Read the model definition and answer for the solid it produces. Units are mm, in the model's axes. A direction names the side the tool comes from. Coordinates: 2 decimals unless noted, no trailing zeros. Loops run counter-clockwise (first coordinate to the right, second up) from the corner with the lowest first, then second, coordinate; pieces in that order, holes last. Notation, with made-up numbers: (77, 50.25) -> (123, 50.25) arc R23 cw to (123, 82.25) -> close; hole circle Ø10 at (88, 37.5). An arc over 180 degrees is marked (long way). Answer as a JSON object with one key per item and string values. Group by question number.
1) Determine the mould class of faces 4 (the face through (70.25, -16, 2)), 5 (the face through (20, -15, 2)), 6 (the face through (110, -15, 2)), 7 (the face through (65, -30, 2)) for opening direction X: released by +X, released by -X, zero draft, split by the parting line, or undercut.
2) Section B-B, the plane y = -7 is taken. Give the vertices of the cut face in (x, z), plus the area to 3 significant figures.
3) Section A-A, the plane y = -18.25 is taken. Give the vertices of the cut face in (x, z).
4) A flat-ended cylindrical pin translates along its axis: P1, Ø1.5, axis at x = 28, z = 1, coming from the -Y side. Find the tip coordinate at first contact, or state that the pin passes through.
5) Section C-C, the plane x = 65 is taken. Give the vertices of the cut face in (y, z).
6) Section D-D, the plane z = 1.75 is taken. Give the vertices of the cut face in (x, y).
7) Consider probe 1 along X at (y, z) = (-24, 1.15); probe 2 along Y at (x, z) = (95.5, 1.35); probe 3 along Y at (x, z) = (89.5, 2.1). Determine where each line is inside the solid, lowest interval first. Write a range as [from, to].
8) Which of the six approach directions +Z, -Z, +X, -X, +Y, -Y give full straight-line access (tool end or side, diameter ignored) to faces 1 (the face through (64, -21, 3)), 2 (the face through (27.05, -23, 1)), 3 (the face through (62.25, -16, 2))?
Autodesk Inventor part; units mm, degrees
ref_plane "YZ Plane" through (0, 0, 0) normal (1, 0, 0) x (0, 1, 0)
ref_plane "XZ Plane" through (0, 0, 0) normal (0, 1, 0) x (-1, 0, 0)
ref_plane "XY Plane" through (0, 0, 0) normal (0, 0, 1) x (1, 0, 0)
sketch "草圖1" plane through (0, 0, 0) normal (0, 0, 1) x (1, 0, 0)
  line L0 (0, 0) -> (130, 0)
  line L1 (130, 0) -> (130, -27)
  line L2 (130, -27) -> (0, -27)
  line L3 (0, -27) -> (0, 0)
  line L4 (27.05, -27) -> (30, -27)
  line L5 (30, -27) -> (30, -16)
  line L6 (30, -16) -> (27.05, -16)
  line L7 (27.05, -16) -> (27.05, -27)
  line L8 (100, -27) -> (102.95, -27)
  line L9 (102.95, -27) -> (102.95, -16)
  line L10 (102.95, -16) -> (100, -16)
  line L11 (100, -16) -> (100, -27)
  line L12 (30, -16) -> (100, -16)
  point P0 (65, -16)
  point P1 (65, -27)
  dimension "d0" = 70
  dimension "d1" = 130
  dimension "d2" = 2.95
  dimension "d3" = 2.95
  dimension "d4" = 11
  dimension "d5" = 27
extrude "擠出1" add sketch "草圖1" along normal blind 3 contours L0 L1 L2 L9 L10 L12 L6 L7 L3 | L5 L12 L11 L2
sketch "草圖4" plane through (0, 0, 3) normal (0, 0, 1) x (1, 0, 0)
  line L0 (0, -27) -> (27.05, -27)
  line L1 (0, -27) -> (130, -27)
  line L2 (130, -27) -> (130, -30)
  line L3 (130, -30) -> (0, -30)
  line L4 (0, -30) -> (0, -27)
  line L5 (100, -27) -> (100, -16)
  line L6 (100, -27) -> (100, -30)
  line L7 (102.95, -16) -> (102.95, -27)
  line L8 (102.95, -27) -> (102.95, -30)
  line L9 (27.05, -27) -> (27.05, -30)
  line L10 (30, -27) -> (100, -27)
  line L11 (30, -27) -> (30, -30)
  line L12 (102.95, -27) -> (130, -27)
  line L13 (110, -27) -> (130, -27)
  line L14 (130, -27) -> (130, 0)
  dimension "d49" = 3
extrude "擠出4" add sketch "草圖4" against normal up to surface (3 mm away) contours L0 L9 L3 L4 | L1 L6 L3 L11 | L1 L2 L3 L8
sketch "草圖5" plane through (0, 0, 3) normal (0, 0, 1) x (1, 0, 0)
  line L0 (130, 0) -> (0, 0)
  line L1 (0, 0) -> (0, -30)
  line L2 (0, -30) -> (27.05, -30)
  line L3 (27.05, -30) -> (27.05, -16)
  line L4 (27.05, -16) -> (30, -16)
  line L5 (30, -16) -> (30, -30)
  line L6 (30, -30) -> (100, -30)
  line L7 (100, -30) -> (100, -16)
  line L8 (100, -16) -> (102.95, -16)
  line L9 (102.95, -16) -> (102.95, -30)
  line L10 (102.95, -30) -> (130, -30)
  line L11 (130, -30) -> (130, 0)
  line L12 (130, -30) -> (102.95, -30)
  line L13 (130, 0) -> (110, 0)
  line L14 (110, 0) -> (110, -30)
  line L15 (110, -30) -> (130, -30)
  line L16 (130, -30) -> (130, 0)
  line L17 (0, -30) -> (0, 0)
  line L18 (0, 0) -> (20, 0)
  line L19 (20, 0) -> (20, -30)
  line L20 (20, -30) -> (0, -30)
  point P0 (130, -15)
  dimension "d33" = 20
  dimension "d51" = 20
extrude "擠出5" cut sketch "草圖5" against normal up to surface (3 mm away) contours L11 L10 L14 L0 | L19 L2 L1 L0
sketch "草圖7" plane through (0, 0, 3) normal (0, 0, 1) x (1, 0, 0)
  line L0 (90.25, -5.137) -> (90.25, -23.137)
  line L1 (90.25, -23.137) -> (92.75, -23.137)
  line L2 (92.75, -23.137) -> (92.75, -5.137)
  line L3 (92.75, -5.137) -> (90.25, -5.137)
  line L4 (100, -30) -> (100, -16)
  line L5 (100, -16) -> (102.95, -16)
  line L6 (90.25, -5.137) -> (90.25, -12.637)
  line L7 (90.25, -12.637) -> (87.75, -12.637)
  line L8 (87.75, -12.637) -> (87.75, -5.137)
  line L9 (87.75, -5.137) -> (90.25, -5.137)
  line L10 (90.25, -15.637) -> (90.25, -23.137)
  line L11 (90.25, -23.137) -> (87.75, -23.137)
  line L12 (87.75, -23.137) -> (87.75, -15.637)
  line L13 (87.75, -15.637) -> (90.25, -15.637)
  line L14 (92.75, -15.137) -> (95.75, -15.137)
  line L15 (95.75, -15.137) -> (95.75, -13.137)
  line L16 (95.75, -13.137) -> (92.75, -13.137)
  line L17 (92.75, -13.137) -> (92.75, -15.137)
  line L18 (102.95, -5.137) -> (102.95, -23.137)
  line L19 (102.95, -23.137) -> (105.45, -23.137)
  line L20 (105.45, -23.137) -> (105.45, -5.137)
  line L21 (105.45, -5.137) -> (102.95, -5.137)
  line L22 (102.95, -16) -> (102.95, -30)
  line L23 (30, -30) -> (100, -30)
  line L24 (62.25, -10.5805) -> (70.25, -10.5805)
  line L25 (70.25, -10.5805) -> (70.25, -20.5805)
  line L26 (70.25, -20.5805) -> (62.25, -20.5805)
  line L27 (62.25, -20.5805) -> (62.25, -10.5805)
  point P0 (0, 0)
  point P1 (91.5, -5.137)
  point P2 (95.75, -14.137)
  point P3 (92.75, -14.137)
  point P4 (66.25, -20.5805)
  dimension "d36" = 7.25
  dimension "d37" = 2.5
  dimension "d38" = 18
  dimension "d40" = 18
  dimension "d41" = 2.5
  dimension "d42" = 7.5
  dimension "d43" = 7.5
  dimension "d44" = 2.5
  dimension "d45" = 2
  dimension "d46" = 3
  dimension "d50" = 6.863
  dimension "d52" = 10
  dimension "d53" = 8
  dimension "d54" = 20
extrude "擠出6" cut sketch "草圖7" against normal up to surface (3 mm away) contours L3 L2 L1 L0 | L0 L7 L8 L9 | L0 L11 L12 L13 | L16 L15 L14 L2 | L24 L25 L26 L27
sketch "草圖9" plane through (0, 0, 3) normal (0, 0, 1) x (1, 0, 0)
  line L0 (102.95, -16) -> (102.95, -30)
  line L1 (102.95, -30) -> (110, -30)
  line L2 (110, -30) -> (110, 0)
  line L3 (110, 0) -> (20, 0)
  line L4 (20, 0) -> (20, -30)
  line L5 (20, -30) -> (27.05, -30)
  line L6 (27.05, -30) -> (27.05, -16)
  line L7 (27.05, -16) -> (30, -16)
  line L8 (30, -16) -> (30, -30)
  line L9 (30, -30) -> (100, -30)
  line L10 (100, -30) -> (100, -16)
  line L11 (100, -16) -> (102.95, -16)
  line L12 (95.75, -15.137) -> (92.75, -15.137)
  line L13 (92.75, -15.137) -> (92.75, -23.137)
  line L14 (92.75, -23.137) -> (87.75, -23.137)
  line L15 (87.75, -23.137) -> (87.75, -15.637)
  line L16 (87.75, -15.637) -> (90.25, -15.637)
  line L17 (90.25, -15.637) -> (90.25, -12.637)
  line L18 (90.25, -12.637) -> (87.75, -12.637)
  line L19 (87.75, -12.637) -> (87.75, -5.137)
  line L20 (87.75, -5.137) -> (92.75, -5.137)
  line L21 (92.75, -5.137) -> (92.75, -13.137)
  line L22 (92.75, -13.137) -> (95.75, -13.137)
  line L23 (95.75, -13.137) -> (95.75, -15.137)
  line L24 (70.25, -20.5805) -> (62.25, -20.5805)
  line L25 (62.25, -20.5805) -> (62.25, -10.5805)
  line L26 (62.25, -10.5805) -> (70.25, -10.5805)
  line L27 (70.25, -10.5805) -> (70.25, -20.5805)
  point P0 (0, 0)
Determined:
{
 "1": {"face 4": "undercut", "face 5": "released by -X", "face 6": "released by +X", "face 7": "zero draft"},
 "2": {"outline": "(20, 0) -> (87.75, 0) -> (87.75, 3) -> (20, 3) -> close; (92.75, 0) -> (110, 0) -> (110, 3) -> (92.75, 3) -> close", "area": "255 mm²"},
 "3": {"outline": "(20, 0) -> (27.05, 0) -> (27.05, 3) -> (20, 3) -> close; (30, 0) -> (62.25, 0) -> (62.25, 3) -> (30, 3) -> close; (70.25, 0) -> (87.75, 0) -> (87.75, 3) -> (70.25, 3) -> close; (92.75, 0) -> (100, 0) -> (100, 3) -> (92.75, 3) -> close; (102.95, 0) -> (110, 0) -> (110, 3) -> (102.95, 3) -> close"},
 "4": {"P1": "y = -16"},
 "5": {"outline": "(-30, 0) -> (-20.58, 0) -> (-20.58, 3) -> (-30, 3) -> close; (-10.58, 0) -> (0, 0) -> (0, 3) -> (-10.58, 3) -> close"},
 "6": {"outline": "(20, -30) -> (27.05, -30) -> (27.05, -16) -> (30, -16) -> (30, -30) -> (100, -30) -> (100, -16) -> (102.95, -16) -> (102.95, -30) -> (110, -30) -> (110, 0) -> (20, 0) -> close; hole (62.25, -20.58) -> (70.25, -20.58) -> (70.25, -10.58) -> (62.25, -10.58) -> close; hole (87.75, -23.14) -> (92.75, -23.14) -> (92.75, -15.14) -> (95.75, -15.14) -> (95.75, -13.14) -> (92.75, -13.14) -> (92.75, -5.14) -> (87.75, -5.14) -> (87.75, -12.64) -> (90.25, -12.64) -> (90.25, -15.64) -> (87.75, -15.64) -> close"},
 "7": {"probe 1": "[20, 27.05], [30, 100], [102.95, 110]", "probe 2": "[-30, -15.14], [-13.14, 0]", "probe 3": "[-30, -23.14], [-15.64, -12.64], [-5.14, 0]"},
 "8": {"face 1": "+Z, +X, -X, +Y, -Y", "face 2": "+Z, -Z, -Y", "face 3": "+Z, -Z"}
}
